Can you work these out from the drawing? Everything is in mm from the part's minimum corner. A direction names the side the tool comes from. Round coordinates to 2 decimals unless told otherwise and drop trailing zeros. Loops run counter-clockwise (first coordinate to the right, second up) from the corner with the lowest first, then second, coordinate; pieces in that order, holes last. Notation, with made-up numbers: (34, 26) - (52, 26) arc R18 ccw to (52, 56) - close; hole circle Ø9 at (56, -28.75). An arc over 180 degrees is marked (long way). Answer as a JSON object with one key per item and string values. Group by question number.
1) I want a section at B-B, the plane z = 10. Please give me the cut outline in (x, y), then the cut area to 3 significant figures.
2) I want a section at D-D, the plane z = 28. Please give me the cut outline in (x, y).
3) I want a section at A-A, the plane y = 26.5. Please give me the cut outline in (x, z), then the cut area to 3 significant figures.
4) Which directions (+Z, -Z, +X, -X, +Y, -Y) give clear straight access to the entire face, cutting with the end or side of a thin tool? Please do the marked faces 5, 6, 7, 8 and 9.
5) Will these pins go through, and if not, where does the flat tip stop? P1, Ø3, axis at x = 24.5, z = 25, coming from the +Y side; P2, Ø15, axis at x = 30, z = 38, coming from the -Y side; P3, Ø4, axis at x = 15, z = 9.5, coming from the +Y side; P4, Ø3.5, axis at x = 43, z = 25, coming from the -Y side.
6) If I drill on line 1 along Z through (x, y) = (13, 28); line 2 along Z through (x, y) = (30, 7); line 3 along X through (y, z) = (7, 25), over which ranges is the centre line in solid material (lowest first)? Write a range as [from, to].
7) If we mould it in two halves opening along X, with no side actions, what happens to the marked faces 1, 2, 3 and 4? For each: pulls with the +X half, pulls with the -X half, needs draft (parallel to the pull), parting line crosses it, or undercut.
8) I want a section at C-C, the plane y = 6.5. Please give me the cut outline in (x, z).
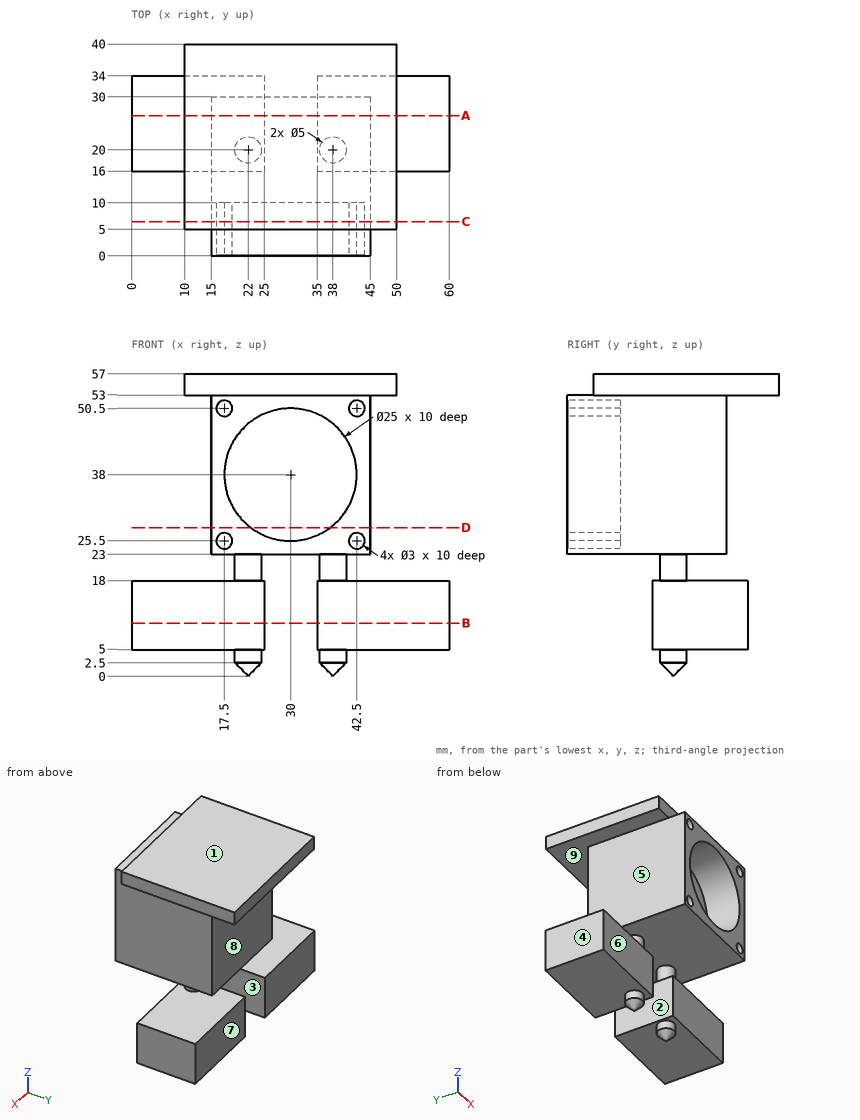
Outcome:
{
 "1": {"outline": "(0, 16) - (25, 16) - (25, 34) - (0, 34) - close; (35, 16) - (60, 16) - (60, 34) - (35, 34) - close", "area": "900 mm^2"},
 "2": {"outline": "(15, 0) - (22.5, 0) - (22.5, 10) - (37.5, 10) - (37.5, 0) - (45, 0) - (45, 30) - (15, 30) - close"},
 "3": {"outline": "(0, 5) - (25, 5) - (25, 18) - (0, 18) - close; (10, 53) - (15, 53) - (15, 23) - (45, 23) - (45, 53) - (50, 53) - (50, 57) - (10, 57) - close; (35, 5) - (60, 5) - (60, 18) - (35, 18) - close", "area": "1,710 mm^2"},
 "4": {"face 5": "-X, +Y, -Y", "face 6": "-Z, +X, -X, -Y", "face 7": "-Z, +X, -X, +Y", "face 8": "+X, -X, +Y", "face 9": "+Y"},
 "5": {"P1": "y = 30", "P2": "y = 10", "P3": "y = 34", "P4": "y = 0"},
 "6": {"line 1": "[5, 18], [53, 57]", "line 2": "[23, 25.5], [50.5, 57]", "line 3": "[15, 16.09], [18.91, 41.09], [43.91, 45]"},
 "7": {"face 1": "needs draft", "face 2": "undercut", "face 3": "undercut", "face 4": "pulls with the -X half"},
 "8": {"outline": "(10, 53) - (15, 53) - (15, 23) - (45, 23) - (45, 53) - (50, 53) - (50, 57) - (10, 57) - close; hole circle Ø3 at (17.5, 25.5); hole circle Ø3 at (17.5, 50.5); hole circle Ø25 at (30, 38); hole circle Ø3 at (42.5, 25.5); hole circle Ø3 at (42.5, 50.5)"}
}
